The figure shows three views and two pictorial views of one solid part (mm, origin at its lowest corner). Answer the questions. A direction names the side the tool comes from. Round coordinates to 2 decimals unless told otherwise and drop trailing zeros. Write each loop counter-clockwise with the first axis right and the second up, starting at its lowest first coordinate (ties: lowest second). Pieces come first, ordered by that corner, then holes. Notation, with made-up numbers: M 16,2 L 71,2 A26 ccw 71,17 Z; hole C 68.5,-11 d3. An arc over 180 degrees is marked long. One line per item, written item: value. Start each with the question number.
Q1. Given pin 1 Ø0.6 at (x, z) = (15.5, 1) entering from -Y; pin 2 Ø8 at (x, y) = (12, 7.5) entering from -Z; pin 3 Ø0.9 at (y, z) = (3.5, 1.5) entering from +X, each flat-ended and moving along its own axis, determine where each tip first touches the part or whether it passes through.
Q2. The mould has two halves that part along X. Classify the marked faces 3, 4 and 5: released by +X, released by -X, zero draft, split by the parting line, or undercut.
Q3. Find section D-D (z = 4.4). Write down the section's boundary in (x, y).
Q4. Consider probe 1 along Z at (x, y) = (14.5, 11.5); probe 2 along Z at (x, y) = (10.75, 12.25); probe 3 along X at (y, z) = (13.25, 4). Determine where each line is inside the solid, lowest interval first.
Q5. Find section A-A (y = 12). Write down the section's boundary in (x, z).
Q6. Find section C-C (y = 2.25). Write down the section's boundary in (x, z), and give its area (3 significant figures).
Q7. Find section B-B (x = 10.5). Write down the section's boundary in (y, z).
Q8. A tool of negligible diameter and unlimited length cuts with its end or side. For the marked faces 1 and 2, from which of +Z, -Z, +X, -X, +Y, -Y can it reach the whole face along a straight path? Write none if from no direction.
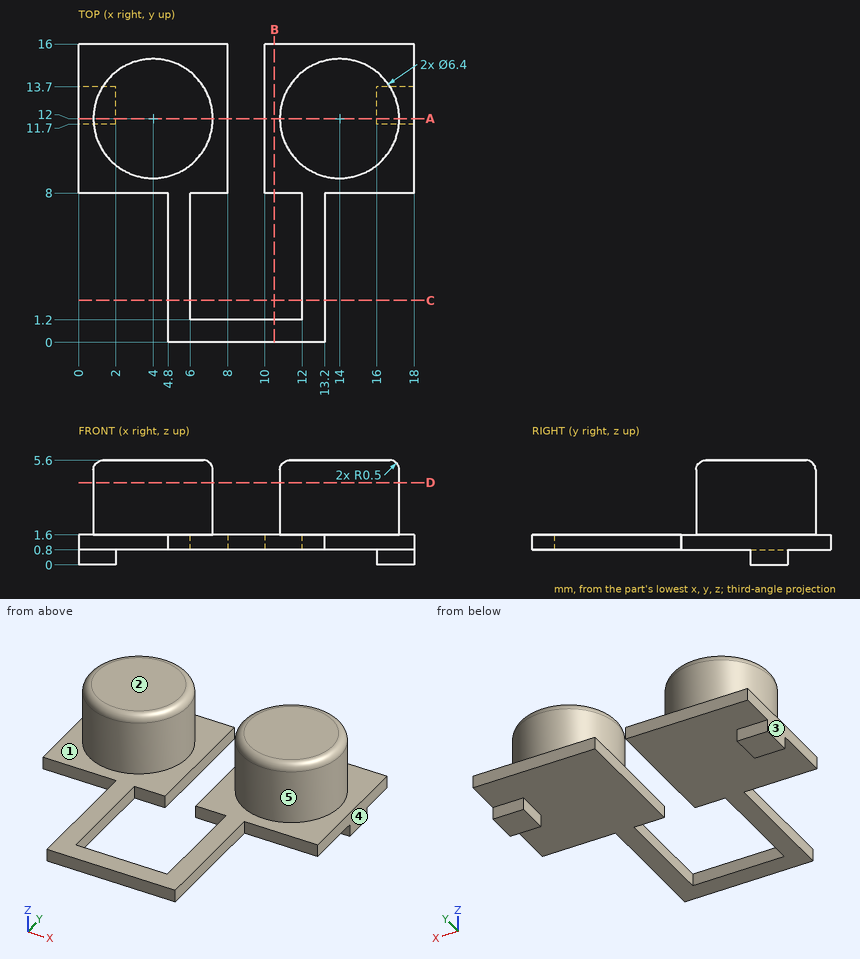
The answers:
1. pin 1: y = 8
1. pin 2: z = 0.8
1. pin 3: x = 13.2
2. face 3: released by -X
2. face 4: released by +X
2. face 5: undercut
3. outline: C 4,12 d6.4; C 14,12 d6.4
4. probe 1: 0.8 to 5.6
4. probe 2: 0.8 to 1.6
4. probe 3: 1.05 to 6.95, 11.05 to 16.95
5. outline: M 0,0 L 2,0 L 2,0.8 L 8,0.8 L 8,1.6 L 7.2,1.6 L 7.2,5.1 A0.5 ccw 6.7,5.6 L 1.3,5.6 A0.5 ccw 0.8,5.1 L 0.8,1.6 L 0,1.6 Z; M 10,0.8 L 16,0.8 L 16,0 L 18,0 L 18,1.6 L 17.2,1.6 L 17.2,5.1 A0.5 ccw 16.7,5.6 L 11.3,5.6 A0.5 ccw 10.8,5.1 L 10.8,1.6 L 10,1.6 Z
6. outline: M 4.8,0.8 L 6,0.8 L 6,1.6 L 4.8,1.6 Z; M 12,0.8 L 13.2,0.8 L 13.2,1.6 L 12,1.6 Z
6. area: 1.92 mm2
7. outline: M 0,0.8 L 1.2,0.8 L 1.2,1.6 L 0,1.6 Z; M 8,0.8 L 16,0.8 L 16,1.6 L 8,1.6 Z
8. face 1: +Z
8. face 2: +Z, +X, -X, +Y, -Y
